Could you check a few things on this drawing? It's one solid part, dimensions in mm from its lowest x, y, z. Give positions to 0.01 mm unless a question says otherwise; leave off trailing zeros. Write each loop counter-clockwise with the first axis right and the second up, starting at its lowest first coordinate (ties: lowest second). Pieces come first, ordered by that corner, then holes.
1. Suppose I cut it at A-A (y = 6). Please give me the cut outline in (x, z), and give its area (3 significant figures).
2. Suppose I cut it at B-B (z = 1.2). Please give me the cut outline in (x, y).
3. I'm going to push a flat-ended pin straight in: pin 1 (3 mm diameter, centred on x = 65, z = 2.5, fed in from -Y). Where does the tip first touch, or does it pass through?
4. If I drill on probe 1 along X at (y, z) = (11, 3.65); probe 2 along Y at (x, z) = (68, 2.15), over which ranges is the centre line in solid material (lowest first)?
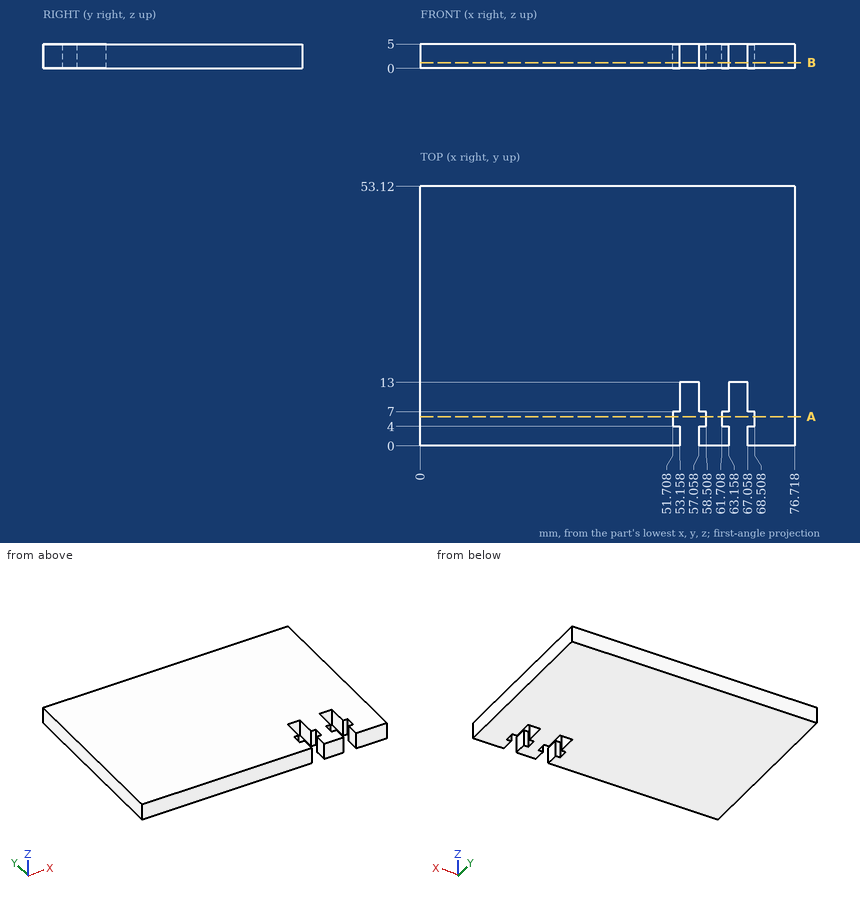
Checks:
1. outline: (0, 0) - (51.71, 0) - (51.71, 5) - (0, 5) - close; (58.51, 0) - (61.71, 0) - (61.71, 5) - (58.51, 5) - close; (68.51, 0) - (76.72, 0) - (76.72, 5) - (68.51, 5) - close
1. area: 316 mm2
2. outline: (0, 0) - (53.16, 0) - (53.16, 4) - (51.71, 4) - (51.71, 7) - (53.16, 7) - (53.16, 13) - (57.06, 13) - (57.06, 7) - (58.51, 7) - (58.51, 4) - (57.06, 4) - (57.06, 0) - (63.16, 0) - (63.16, 4) - (61.71, 4) - (61.71, 7) - (63.16, 7) - (63.16, 13) - (67.06, 13) - (67.06, 7) - (68.51, 7) - (68.51, 4) - (67.06, 4) - (67.06, 0) - (76.72, 0) - (76.72, 53.12) - (0, 53.12) - close
3. pin 1: stops at y = 13
4. probe 1: x = 0 to 53.16, 57.06 to 63.16, 67.06 to 76.72
4. probe 2: y = 0 to 4, 7 to 53.12
